Could you check a few things on this model? Use its own coordinates, in mm. Round coordinates to 2 decimals unless told otherwise and drop trailing zeros. Order: outer loops, then holes, each group sorted by start corner. A loop starts at its lowest first (then second) coordinate and runs counter-clockwise, first axis right, second up. Notation, with made-up numbers: (-22.75, 38) -> (3.25, 38) arc R11 ccw to (3.25, 44) -> close; hole circle Ø2 at (59, 36). An arc over 180 degrees is marked (long way). One line per question, with ' | ' between items.
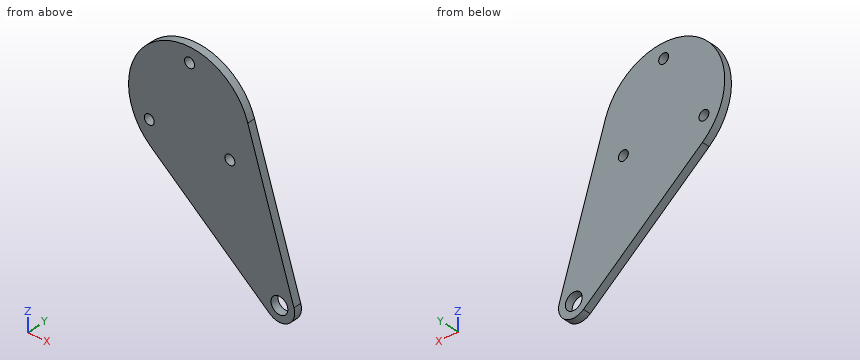
```python
from build123d import *

# Parameters (mm, degrees)
F0_R     = 5.5
F0_R_2   = 3.25
F1_DEPTH = 5


with BuildPart() as f1:
    # F0 (on Front) → F1 (new body)
    with BuildSketch(Plane.XZ):
        with BuildLine():
            Line((68.416541, -84.14495), (38.15498, 12.008228))
            ThreePointArc((38.15498, 12.008228), (-22.392908, 33.144497), (-25.379985, -30.916927))
            Line((-25.379985, -30.916927), (52.5328, -94.876239))
            ThreePointArc((52.5328, -94.876239), (64.476024, -95.433131), (68.416541, -84.14495))
        make_face()
        with Locations((58.877797, -87.147007)):
            Circle(F0_R, mode=Mode.SUBTRACT)
        with Locations((-26.413775, -15.25)):
            Circle(F0_R_2, mode=Mode.SUBTRACT)
        with Locations((0, 30.5)):
            Circle(F0_R_2, mode=Mode.SUBTRACT)
        with Locations((26.413775, -15.25)):
            Circle(F0_R_2, mode=Mode.SUBTRACT)
    extrude(amount=F1_DEPTH)


solid = f1.part
```
1. I want a section at A-A on z = 30.5. List the corners of the cut face in (x, y) for me, and give its area (3 significant figures).
From the geometry:
outline: (-25.88, -5) -> (-3.25, -5) -> (-3.25, 0) -> (-25.88, 0) -> close; (3.25, -5) -> (25.88, -5) -> (25.88, 0) -> (3.25, 0) -> close | area: 226 mm²
2. I want a section at B-B on y = -1.25. List the corners of the cut face in (x, z) for me, and give its area (3 significant figures).
From the geometry:
outline: (-25.38, -30.92) -> (52.53, -94.88) arc R10 ccw to (68.42, -84.14) -> (38.15, 12.01) arc R40 ccw (long way) to start; hole circle Ø6.5 at (-26.41, -15.25); hole circle Ø6.5 at (0, 30.5); hole circle Ø6.5 at (26.41, -15.25); hole circle Ø11 at (58.88, -87.15) | area: 7,950 mm²
3. I want a section at D-D on x = -14. List the corners of the cut face in (y, z) for me, and give its area (3 significant figures).
From the geometry:
outline: (-5, -40.26) -> (0, -40.26) -> (0, 37.47) -> (-5, 37.47) -> close | area: 389 mm²
4. I want a section at C-C on x = 0. List the corners of the cut face in (y, z) for me, and give its area (3 significant figures).
From the geometry:
outline: (-5, -51.75) -> (0, -51.75) -> (0, 27.25) -> (-5, 27.25) -> close; (-5, 33.75) -> (0, 33.75) -> (0, 40) -> (-5, 40) -> close | area: 426 mm²
5. I'm going to push a flat-ended pin straight in: pin 1 (1.5 mm diameter, centred on x = -3.5, y = -2, fed in from +Z). Where does the tip first touch, or does it pass through?
From the geometry:
pin 1: stops at z = 39.91
6. I need wall thicknesses on probe 1 along X at (y, z) = (-3.6, 32.5); probe 2 along Z at (x, y) = (-28.5, -3.9); probe 3 along Z at (x, y) = (0, -3.4). Which ranges of each line are inside material? Lowest first, please.
From the geometry:
probe 1: x = -23.32 to -2.56, 2.56 to 23.32 | probe 2: z = -28.07 to -17.74, -12.76 to 28.07 | probe 3: z = -51.75 to 27.25, 33.75 to 40
